For this review, take the finished solid that the model builds, in its own axes (mm). A direction names the side the tool comes from. Coordinates: 2 decimals unless noted, no trailing zeros. Order: outer loops, then holes, each group sorted by start corner. A loop starts at its lowest first (then second) coordinate and runs counter-clockwise, first axis right, second up. Notation, with made-up numbers: M 78.5,22.25 L 126.5,22.25 A13 cw 126.5,30.25 Z; hole C 58.25,16 d6. An arc over 180 degrees is marked long. Use CSV: the item, a comma, the result in double quotes.
```python
from build123d import *

# Parameters (mm, degrees)
F0_W      = 8.75
F0_H      = 8.75
F1_DEPTH  = 7.5
F2_T      = -1.5
F4_DEPTH  = 7.5
F6_DEPTH  = 3
F7_R      = 3.25
F8_DEPTH  = 32.25
F9_R      = 3.25
F10_DEPTH = 32.25


with BuildPart() as f1:
    # F0 (on Top) → F1 (new body)
    with BuildSketch(Plane.XY):
        Polygon((25, 0), (25, 8.75), (8.75, 8.75), (0, 8.75), (0, 0), align=None)
        Polygon((25, -8.75), (25, 0), (0, 0), (0, -25), (8.75, -25), (8.75, -8.75), align=None)
        with Locations((-4.375, 4.375)):
            Rectangle(F0_W, F0_H)
        Polygon((0, -25), (0, 0), (-8.75, 0), (-8.75, -8.75), (-8.75, -25), align=None)
    extrude(amount=F1_DEPTH)

    # F2
    f2_openings = [f1.faces().sort_by_distance(p)[0] for p in [
        (5.484375, -5.484375, 7.5),
    ]]
    offset(amount=F2_T, openings=f2_openings, kind=Kind.INTERSECTION)

    # F3 (on face) → F4 (join, through all)
    with BuildSketch(Plane.XY.offset(7.5)):
        Polygon((-4.4215728753, 7.25), (-7.25, 7.25), (-7.25, 4.4215728753), align=None)
        Polygon((11.5784271247, -8.75), (8.75, -8.75), (8.75, -11.5784271247), align=None)
        Polygon((23.5, 7.25), (20.6715728753, 7.25), (23.5, 4.4215728753), align=None)
        Polygon((-4.4215728753, -23.5), (-7.25, -20.6715728753), (-7.25, -23.5), align=None)
    extrude(amount=-F4_DEPTH)

    # F5 (on face) → F6 (cut)
    with BuildSketch(Plane.XY.offset(7.5)):
        with BuildLine():
            ThreePointArc((-6.3661165235, 6.3661165235), (-6.20353696, 6.6094340351), (-6.1464466094, 6.8964466094))
            ThreePointArc((-6.1464466094, 6.8964466094), (-7.5893562588, 7.1834591837), (-6.3661165235, 6.3661165235))
        make_face()
        with BuildLine():
            ThreePointArc((22.6161165235, 6.3661165235), (23.4334591837, 6.20353696), (23.8964466094, 6.8964466094))
            ThreePointArc((23.8964466094, 6.8964466094), (22.8594340351, 7.5893562588), (22.6161165235, 6.3661165235))
        make_face()
        with BuildLine():
            ThreePointArc((9.6338834765, -9.6338834765), (9.79646304, -9.3905659649), (9.8535533906, -9.1035533906))
            ThreePointArc((9.8535533906, -9.1035533906), (8.4106437412, -8.8165408163), (9.6338834765, -9.6338834765))
        make_face()
        with BuildLine():
            ThreePointArc((-6.3661165235, -22.6161165235), (-7.5893562588, -23.4334591837), (-6.1464466094, -23.1464466094))
            ThreePointArc((-6.1464466094, -23.1464466094), (-6.20353696, -22.8594340351), (-6.3661165235, -22.6161165235))
        make_face()
    extrude(amount=-F6_DEPTH, mode=Mode.SUBTRACT)

    # F7 (on face) → F8 (cut, through all)
    with BuildSketch(Plane.XZ.offset(25)):
        with Locations((0, 7.5)):
            Circle(F7_R)
    extrude(amount=-F8_DEPTH, mode=Mode.SUBTRACT)

    # F9 (on face) → F10 (cut, through all)
    with BuildSketch(Plane.YZ.offset(25)):
        with Locations((0, 7.5)):
            Circle(F9_R)
    extrude(amount=-F10_DEPTH, mode=Mode.SUBTRACT)


solid = f1.part
```
Item 1: Add section B-B on x = 0. State the section outline as (y, z) points.
Solutions:
outline,"M -25,0 L 8.75,0 L 8.75,7.5 L 7.25,7.5 L 7.25,1.5 L -23.5,1.5 L -23.5,4.25 L -25,4.25 Z"
Item 2: Add section A-A on z = 5.5. State the section outline as (x, y) points, and give its area (3 significant figures).
Solutions:
outline,"M -8.75,-25 L -2.56,-25 L -2.56,-23.5 L -4.42,-23.5 L -7.25,-20.67 L -7.25,4.42 L -4.42,7.25 L 20.67,7.25 L 23.5,4.42 L 23.5,2.56 L 25,2.56 L 25,8.75 L -8.75,8.75 Z; M 2.56,-25 L 8.75,-25 L 8.75,-11.58 L 11.58,-8.75 L 25,-8.75 L 25,-2.56 L 23.5,-2.56 L 23.5,-7.25 L 7.25,-7.25 L 7.25,-23.5 L 2.56,-23.5 Z; hole C -6.9,-23.15 d1.5; hole C -6.9,6.9 d1.5; hole C 9.1,-9.1 d1.5; hole C 23.15,6.9 d1.5"
area,"187 mm^2"
Item 3: To check wall thickness, follow line 1 along X through (y, z) = (4, 2.25); line 2 along X through (y, z) = (7.5, 5); line 3 along Y through (x, z) = (3.5, 5). State the ranges of each line that lie inside material, in increasing order. Write a range as [from, to].
Solutions:
line 1,"[-8.75, -7.25], [23.5, 25]"
line 2,"[-8.75, -7.34], [-6.45, 22.7], [23.59, 25]"
line 3,"[-25, -23.5], [7.25, 8.75]"
Item 4: Draft analysis for pull direction Y (two halves, no side actions). For faces 1 (the face through (-5.816, -22.106, 4.542)), 2 (the face through (10.144, -10.184, 3.802)), 3 (the face through (-8.75, -8, 4)), 4 (the face through (8, 8.75, 4)), state which applies: released by +Y, released by -Y, zero draft, split by the parting line, or undercut.
Solutions:
face 1,"undercut"
face 2,"released by -Y"
face 3,"zero draft"
face 4,"released by +Y"
Item 5: Add section D-D on z = 2.25. State the section outline as (x, y) points, and give its area (4 significant figures).
Solutions:
outline,"M -8.75,-25 L 8.75,-25 L 8.75,-11.58 L 11.58,-8.75 L 25,-8.75 L 25,8.75 L -8.75,8.75 Z; hole M -7.25,-20.67 L -4.42,-23.5 L 7.25,-23.5 L 7.25,-7.25 L 23.5,-7.25 L 23.5,4.42 L 20.67,7.25 L -4.42,7.25 L -7.25,4.42 Z"
area,"209.5 mm^2"
Item 6: For faces 5 (the face through (-5.856, 5.816, 4.542)), 6 (the face through (8.75, -18, 4)), 7 (the face through (24.26, -0.07, 4.25)), 8 (the face through (-0.07, -24.26, 4.25)), list the 3-axis set-ups (+Z, -Z, +X, -X, +Y, -Y) from which the entire face can be reached by the end or side of a thin tool; tool diameter is ignored.
Solutions:
face 5,"+Z"
face 6,"+Z, -Z, +X, -Y"
face 7,"+Z, +X"
face 8,"+Z, -Y"
Item 7: Add section C-C on y = -5.5. State the section outline as (x, z) points, and give its area (3 significant figures).
Solutions:
outline,"M -8.75,0 L 25,0 L 25,7.5 L 23.5,7.5 L 23.5,1.5 L -7.25,1.5 L -7.25,7.5 L -8.75,7.5 Z"
area,"68.6 mm^2"
Item 8: Clearance check with flat-ended pins moving along their axes: pin 1 Ø1.5 at (x, z) = (17, 4.5) entering from -Y; pin 2 Ø6 at (x, y) = (7, 2.5) entering from +Z; pin 3 Ø0.9 at (x, y) = (9.1, -9.1) entering from +Z. State where each tip first meets the part, or that it passes through.
Solutions:
pin 1,"y = -8.75"
pin 2,"z = 1.5"
pin 3,"z = 4.5"
